Geometry check sheet. Reference: the model listing, model coordinates, mm. A direction names the side the tool comes from. Round coordinates to 2 decimals unless told otherwise and drop trailing zeros. Order: outer loops, then holes, each group sorted by start corner. A loop starts at its lowest first (then second) coordinate and runs counter-clockwise, first axis right, second up. Notation, with made-up numbers: (58.25, -37) - (76.25, -37) arc R12 cw to (76.25, -30) - close; hole circle Ø10 at (-2.75, 63.25). An arc over 180 degrees is marked (long way). Write each question's results on one line, items separated by ' | '.
```python
from build123d import *

# Parameters (mm, degrees)
PAD001_DEPTH    = 2
SKETCH001_W     = 4.83
SKETCH001_H     = 12.7
POCKET_DEPTH    = 2
SKETCH006_W     = 4.83
SKETCH006_H     = 5.08
POCKET001_DEPTH = 2
SKETCH007_W     = 4.83
SKETCH007_H     = 5.08
POCKET002_DEPTH = 2
SKETCH029_R     = 1.1
POCKET011_DEPTH = 2
SKETCH030_R     = 1.1
POCKET012_DEPTH = 2


with BuildPart() as part:
    # Sketch → Pad001 (new body)
    with BuildSketch(Plane.XY):
        Polygon((-8.666667, 13), (8.666667, 13), (8.666667, 11), (26, 11), (26, 3.666667), (28, 3.666667), (28, -3.666667), (26, -3.666667), (26, -11), (8.666667, -11), (8.666667, -13), (-8.666667, -13), (-8.666667, -11), (-26, -11), (-26, -3.666667), (-28, -3.666667), (-28, 3.666667), (-26, 3.666667), (-26, 11), (-8.666667, 11), align=None)
    extrude(amount=PAD001_DEPTH)

    # Sketch001 (on Face22 of Pad001) → Pocket (cut)
    with BuildSketch(Plane.XY.offset(2)):
        with Locations((18.25, 3)):
            Rectangle(SKETCH001_W, SKETCH001_H)
    extrude(amount=-POCKET_DEPTH, mode=Mode.SUBTRACT)

    # Sketch006 (on Face5 of Pocket) → Pocket001 (cut)
    with BuildSketch(Plane.XY.offset(2)):
        with Locations((-18, 0)):
            Rectangle(SKETCH006_W, SKETCH006_H)
    extrude(amount=-POCKET001_DEPTH, mode=Mode.SUBTRACT)

    # Sketch007 (on Face5 of Pocket001) → Pocket002 (cut)
    with BuildSketch(Plane.XY.offset(2)):
        with Locations((-18, -7)):
            Rectangle(SKETCH007_W, SKETCH007_H)
    extrude(amount=-POCKET002_DEPTH, mode=Mode.SUBTRACT)

    # Sketch029 (on Face5 of Pocket002) → Pocket011 (cut)
    with BuildSketch(Plane.XY.offset(2)):
        with Locations((-22, 7)):
            Circle(SKETCH029_R)
    extrude(amount=-POCKET011_DEPTH, mode=Mode.SUBTRACT)

    # Sketch030 (on Face5 of Pocket011) → Pocket012 (cut)
    with BuildSketch(Plane.XY.offset(2)):
        with Locations((22, -7)):
            Circle(SKETCH030_R)
    extrude(amount=-POCKET012_DEPTH, mode=Mode.SUBTRACT)


with BuildPart() as part_1:
    # Body001 placement: moved
    add(part.part.moved(Location((-26, -11, 14))))


solid = part_1.part
```
(1) Section check A-A (x = -48). Record the cut outline in (y, z).
Answers follow:
outline: (-22, 14) - (-5.1, 14) - (-5.1, 16) - (-22, 16) - close; (-2.9, 14) - (0, 14) - (0, 16) - (-2.9, 16) - close
(2) Depth check by flat-ended pin: pin 1 Ø1 at (x, z) = (-43.5, 15) entering from -Y; pin 2 Ø1 at (y, z) = (-18.5, 14.5) entering from +X; pin 3 Ø1 at (y, z) = (-23, 15.5) entering from -X; pin 4 Ø1.8 at (x, y) = (-4, -18) entering from +Z. Enter the tip coordinate at first touch or a pass-through.
Answers follow:
pin 1: y = -22 | pin 2: x = 0 | pin 3: x = -34.67 | pin 4: through
(3) Access from +Z, -Z, +X, -X, +Y, -Y to the whole of each face (thin tool, end or side, straight path). Record for faces 5 (the face through (-46.415, -11, 15)), 6 (the face through (-9, 0, 15)), 7 (the face through (-43, -22, 15)), 8 (the face through (-52, -4, 15)).
Answers follow:
face 5: +Z, -Z | face 6: +Z, -Z, +X, +Y | face 7: +Z, -Z, -X, -Y | face 8: +Z, -Z, -X, +Y
(4) Section check C-C (z = 15). Give the number of separate pieces and of enclosed holes in the cut face, then the cut area to 3 significant figures.
Answers follow:
separate pieces: 1 | enclosed holes: 5 | area: 1,120 mm²
(5) Material ranges on line 1 (X direction, y = -12, z = 14.35) (3 decimals); line 2 (Y direction, x = -48, z = 15.4); line 3 (Y direction, x = -4, z = 15.15), recorded low to high.
Answers follow:
line 1: -54 to -46.415, -41.585 to -10.165, -5.335 to 2 | line 2: -22 to -5.1, -2.9 to 0 | line 3: -22 to -19.1, -16.9 to 0
(6) Section check B-B (y = -11.5). Record the cut outline in (x, z) (3 decimals).
Answers follow:
outline: (-54, 14) - (-46.415, 14) - (-46.415, 16) - (-54, 16) - close; (-41.585, 14) - (-10.165, 14) - (-10.165, 16) - (-41.585, 16) - close; (-5.335, 14) - (2, 14) - (2, 16) - (-5.335, 16) - close
(7) Section check D-D (y = -4). Record the cut outline in (x, z) (3 decimals).
Answers follow:
outline: (-52, 14) - (-49.1, 14) - (-49.1, 16) - (-52, 16) - close; (-46.9, 14) - (-10.165, 14) - (-10.165, 16) - (-46.9, 16) - close; (-5.335, 14) - (0, 14) - (0, 16) - (-5.335, 16) - close
(8) Draft check along Y on faces 1 (the face through (-44, -15.46, 15)), 2 (the face through (-41.585, -11, 15)), 3 (the face through (-26, 2, 15)), 4 (the face through (-17.333, -23, 15)). Enter one of: released by +Y, released by -Y, zero draft, split by the parting line, or undercut.
Answers follow:
face 1: undercut | face 2: undercut | face 3: released by +Y | face 4: zero draft
